Check sheet for the modelled part. Datum: model origin and axes. Units: mm. A direction names the side the tool comes from. Round coordinates to 2 decimals unless told otherwise and drop trailing zeros. Write each loop counter-clockwise with the first axis right and the second up, starting at its lowest first coordinate (ties: lowest second). Pieces come first, ordered by that corner, then holes.
Item 1: Cross-section at B-B on y = -17.5. Enter the section's corners in (x, z), plus the area to 3 significant figures.
Item 2: Material ranges on line 1 (Y direction, x = 16, z = -8); line 2 (X direction, y = -10.75, z = -3); line 3 (Z direction, x = 26.5, y = -11.5), recorded low to high.
Item 3: Release check for a two-part mould opening along Y. For faces 1 (the flat face through (0.43, -10.72, -10.14)), 2 (the flat face through (18.8, -12, -3)), 3 (the cylindrical face through (-24.716, -12.421, -3.895)), 4 (the flat face through (30.8, -16, -7)) record: +Y half, -Y half, draft (parallel to the pull), parting line (faces both ways), or undercut.
Item 4: Tool access check on faces 5 (the flat face through (-18.8, -12, -3)), 6 (the flat face through (0, -21, -10)), 7 (the flat face through (18.8, -18, -7)). Record the directions out of +Z, -Z, +X, -X, +Y, -Y that give a thin tool (end or side, any length) a straight path to the whole face; none if there is none.
Item 5: Cross-section at D-D on x = -14.5. Enter the section's corners in (y, z).
Item 6: Cross-section at A-A on x = 20. Enter the section's corners in (y, z).
Item 7: Go/stop test with flat-tipped pins: pin 1 Ø4 at (x, z) = (-14, -18.5) entering from +Y; pin 2 Ø2 at (y, z) = (-17.5, -7.05) entering from -X; pin 3 Ø2 at (y, z) = (-11.5, -3.05) entering from +X. Record where each tip stops, or that it passes through.
from build123d import *

# Parameters (mm, degrees)
SKETCH1_R               = 2.15
BOSS_EXTRUDE1_DEPTH     = 31.3
CUT_EXTRUDE1_REACH      = 47.396
SKETCH2_W               = 57.6
SKETCH2_H               = 12
CUT_EXTRUDE3_DEPTH      = 70.302687538
CUT_EXTRUDE4_DEPTH      = 40.979432212
CUT_EXTRUDE4_DEPTH_BACK = 40.979432212
SKETCH9_W               = 62.6
SKETCH9_H               = 52.1
SKETCH9_W_2             = 61.6
SKETCH9_H_2             = 50.1
SKETCH10_R              = 1.25
CUT_EXTRUDE5_DEPTH      = 12
CUT_EXTRUDE6_START      = -12
SKETCH11_R              = 1.25
CUT_EXTRUDE6_DEPTH      = 12


with BuildPart() as part:
    # Sketch1 → Boss-Extrude1 (new, symmetric)
    with BuildSketch(Plane(origin=(0, 0, 0), x_dir=(0, 0, -1), z_dir=(1, 0, 0))):
        with BuildLine():
            Line((-4.25, 0), (-4.25, -4))
            ThreePointArc((-4.25, -4), (-4.105356672, -4.642657212), (-3.699322277, -5.161372987))
            Line((-3.699322277, -5.161372987), (-2.000677723, -6.549868444))
            ThreePointArc((-2.000677723, -6.549868444), (-1.594643328, -7.068584218), (-1.45, -7.71124143))
            Line((-1.45, -7.71124143), (-1.45, -21))
            Line((-1.45, -21), (21.05, -21))
            Line((21.05, -21), (11.593870957, -13.612062296))
            Line((11.593870957, -13.612062296), (3.79776528, 1.907741826))
            ThreePointArc((3.79776528, 1.907741826), (-0.980305452, 4.135396138), (-4.25, 0))
        make_face()
        Circle(SKETCH1_R, mode=Mode.SUBTRACT)
    extrude(amount=BOSS_EXTRUDE1_DEPTH, both=True)

    # Cut-Extrude1: up to this plane
    cut_extrude1_end = Plane(origin=(31.3, -13.612062296, -11.593870957), z_dir=(0, -0.44888042970734693, 0.8935918306619346))
    # Sketch2 → Cut-Extrude1 (cut, up to the surface)
    with BuildSketch(Plane.XY.offset(4.25), mode=Mode.PRIVATE) as cut_extrude1_sk1:
        with Locations((0, -1.75)):
            Rectangle(SKETCH2_W, SKETCH2_H)
    cut_extrude1_tool1 = split(extrude(cut_extrude1_sk1.sketch, amount=-CUT_EXTRUDE1_REACH, mode=Mode.PRIVATE), bisect_by=cut_extrude1_end, keep=Keep.BOTH, mode=Mode.PRIVATE)
    add(cut_extrude1_tool1.solids().sort_by_distance((0, -1.75, 4.25))[0], mode=Mode.SUBTRACT)

    # Sketch8 → Cut-Extrude3 (cut, through all)
    with BuildSketch(Plane(origin=(31.3, 0, 0), x_dir=(0, 0, -1), z_dir=(1, 0, 0))):
        with BuildLine():
            Line((-1.45, -7.71124143), (8.649165161, -7.75))
            Line((8.649165161, -7.75), (3.79776528, 1.907741826))
            ThreePointArc((3.79776528, 1.907741826), (-0.980305452, 4.135396138), (-4.25, 0))
            Line((-4.25, 0), (-4.25, -4))
            ThreePointArc((-4.25, -4), (-4.105356672, -4.642657212), (-3.699322277, -5.161372987))
            Line((-3.699322277, -5.161372987), (-2.000677723, -6.549868444))
            ThreePointArc((-2.000677723, -6.549868444), (-1.594643328, -7.068584218), (-1.45, -7.71124143))
        make_face()
    extrude(amount=-CUT_EXTRUDE3_DEPTH, mode=Mode.SUBTRACT)

    # Sketch9 → Cut-Extrude4 (cut, two sides: drawn at the far end of the back side and taken through both)
    with BuildSketch(Plane(origin=(0, -7.75, 0), x_dir=(1, 0, 0), z_dir=(0, 1, 0)).offset(-CUT_EXTRUDE4_DEPTH_BACK)):
        Rectangle(SKETCH9_W, SKETCH9_H)
        Rectangle(SKETCH9_W_2, SKETCH9_H_2, mode=Mode.SUBTRACT)
    extrude(amount=CUT_EXTRUDE4_DEPTH + CUT_EXTRUDE4_DEPTH_BACK, mode=Mode.SUBTRACT)

    # Sketch10 → Cut-Extrude5 (cut)
    with BuildSketch(Plane(origin=(30.8, 0, 0), x_dir=(0, 0, -1), z_dir=(1, 0, 0))):
        with Locations(Location((3.05, -11.5, 0), (0, 0, 90))):
            Circle(SKETCH10_R)
        with Locations(Location((7.05, -17.5, 0), (0, 0, 90))):
            Circle(SKETCH10_R)
    extrude(amount=-CUT_EXTRUDE5_DEPTH, mode=Mode.SUBTRACT)

    # Sketch11 → Cut-Extrude6 (cut)
    with BuildSketch(Plane.ZY.offset(30.8).offset(CUT_EXTRUDE6_START)):
        with Locations(Location((-7.05, -17.5, 0), (0, 0, 90))):
            Circle(SKETCH11_R)
        with Locations(Location((-3.05, -11.5, 0), (0, 0, 90))):
            Circle(SKETCH11_R)
    extrude(amount=CUT_EXTRUDE6_DEPTH, mode=Mode.SUBTRACT)


solid = part.part
Response values:
1. outline: (-30.8, -16.57) - (30.8, -16.57) - (30.8, -8.3) - (18.8, -8.3) - (18.8, -5.8) - (30.8, -5.8) - (30.8, 1.45) - (-30.8, 1.45) - (-30.8, -5.8) - (-18.8, -5.8) - (-18.8, -8.3) - (-30.8, -8.3) - close
1. area: 1,050 mm2
2. line 1: y = -21 to -7.75
2. line 2: x = -18.8 to 18.8
2. line 3: z = -10.53 to -4.3, -1.8 to 1.45
3. face 1: +Y half
3. face 2: undercut
3. face 3: undercut
3. face 4: draft
4. face 5: -X
4. face 6: +Z, -Z, +X, -X, -Y
4. face 7: +X
5. outline: (-21, -21.05) - (-13.61, -11.59) - (-7.75, -8.65) - (-7.75, 1.45) - (-21, 1.45) - close
6. outline: (-21, -21.05) - (-13.61, -11.59) - (-7.75, -8.65) - (-7.75, 1.45) - (-21, 1.45) - close; hole circle Ø2.5 at (-17.5, -7.05); hole circle Ø2.5 at (-11.5, -3.05)
7. pin 1: stops at y = -17.45
7. pin 2: stops at x = -18.8
7. pin 3: stops at x = 18.8
